Here's how the part is built. I have some questions about the finished solid (model axes, mm). Face numbers are marked on the shaded views. A direction names the side the tool comes from. Round coordinates to 2 decimals unless told otherwise and drop trailing zeros. Loops run counter-clockwise (first coordinate to the right, second up) from the corner with the lowest first, then second, coordinate; pieces in that order, holes last. Notation, with made-up numbers: M 6.25,43 L 16.25,43 A25 cw 16.25,78 Z; hole C 3.5,65.25 d5. An arc over 180 degrees is marked long. Answer as CSV lines item,"result".
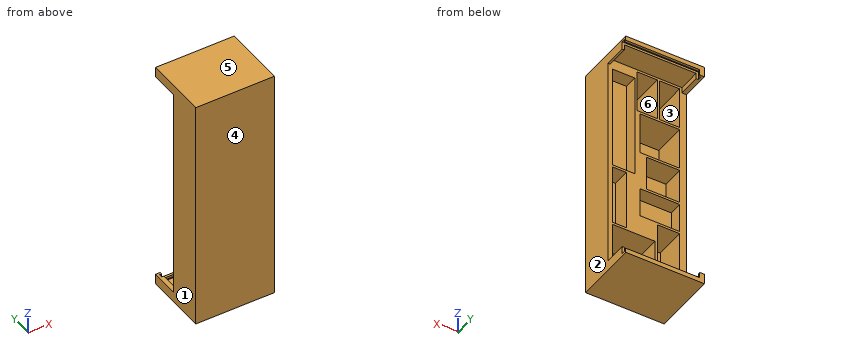
```python
from build123d import *

# Parameters (mm, degrees)
SKETCH1_4_W          = 19.5
SKETCH1_4_H          = 56.2
BOSS_EXTRUDE3_DEPTH  = 2
SKETCH1_5_W          = 12.1
SKETCH1_5_H          = 52.7
BOSS_EXTRUDE4_DEPTH  = 13.8
SKETCH1_W            = 19.5
SKETCH1_H            = 91.3
BOSS_EXTRUDE5_DEPTH  = 17.3
SKETCH1_8_W          = 34.6
SKETCH1_8_H          = 25.8
BOSS_EXTRUDE7_DEPTH  = 17.2
SKETCH1_9_W          = 28.8
SKETCH1_9_H          = 30.5
BOSS_EXTRUDE8_DEPTH  = 9.7
SKETCH1_10_W         = 17.5
SKETCH1_10_H         = 36.9
SKETCH1_10_W_2       = 28.8
SKETCH1_10_H_2       = 30.5
SKETCH1_10_W_3       = 34.6
SKETCH1_10_H_3       = 25.8
SKETCH1_10_W_4       = 19.5
SKETCH1_10_H_4       = 56.2
SKETCH1_10_W_5       = 12.1
SKETCH1_10_H_5       = 52.7
SKETCH1_10_W_6       = 37
SKETCH1_10_H_6       = 39.55
BOSS_EXTRUDE9_DEPTH  = 28.791978309
BOSS_EXTRUDE10_DEPTH = 48.4
BOSS_EXTRUDE11_DEPTH = 53.4
BOSS_EXTRUDE12_DEPTH = 2
SKETCH1_13_W         = 68.5
SKETCH1_13_H         = 206.3
BOSS_EXTRUDE13_DEPTH = 2


with BuildPart() as part:
    # Sketch1_4 → Boss-Extrude3 (new body)
    with BuildSketch(Plane(origin=(0, 0, 0), x_dir=(1, 0, 0), z_dir=(0, 1, 0))):
        with Locations((-18.5, 69.05)):
            Rectangle(SKETCH1_4_W, SKETCH1_4_H)
    extrude(amount=BOSS_EXTRUDE3_DEPTH)



with BuildPart() as body_2:
    # Sketch1_5 → Boss-Extrude4 (new body)
    with BuildSketch(Plane(origin=(0, 0, 0), x_dir=(1, 0, 0), z_dir=(0, 1, 0))):
        with Locations((24.2, 29.25)):
            Rectangle(SKETCH1_5_W, SKETCH1_5_H)
    extrude(amount=BOSS_EXTRUDE4_DEPTH)


with BuildPart() as body_3:
    # Sketch1 → Boss-Extrude5 (new body)
    with BuildSketch(Plane(origin=(0, 0, 0), x_dir=(1, 0, 0), z_dir=(0, 1, 0))):
        with Locations((20.5, -44.75)):
            Rectangle(SKETCH1_W, SKETCH1_H)
    extrude(amount=BOSS_EXTRUDE5_DEPTH)


with BuildPart() as body_4:
    # Sketch1_8 → Boss-Extrude7 (new body)
    with BuildSketch(Plane(origin=(0, 0, 0), x_dir=(1, 0, 0), z_dir=(0, 1, 0))):
        with Locations((-10.95, 26.05)):
            Rectangle(SKETCH1_8_W, SKETCH1_8_H)
    extrude(amount=BOSS_EXTRUDE7_DEPTH)


with BuildPart() as body_5:
    # Sketch1_9 → Boss-Extrude8 (new body)
    with BuildSketch(Plane(origin=(0, 0, 0), x_dir=(1, 0, 0), z_dir=(0, 1, 0))):
        with Locations((-13.85, -4.1)):
            Rectangle(SKETCH1_9_W, SKETCH1_9_H)
    extrude(amount=BOSS_EXTRUDE8_DEPTH)


with BuildPart() as part_1:
    add(part.part)

    add(body_2.part)  # Boss-Extrude9 merges body 2

    add(body_3.part)  # Boss-Extrude9 merges body 3

    add(body_4.part)  # Boss-Extrude9 merges body 4

    add(body_5.part)  # Boss-Extrude9 merges body 5
    # Sketch1_10 → Boss-Extrude9 (add)
    with BuildSketch(Plane(origin=(0, 0, 0), x_dir=(1, 0, 0), z_dir=(0, 1, 0))):
        Polygon((34.25, -94.15), (34.25, 94.15), (32.25, 94.15), (32.25, 99.15), (-30.25, 99.15), (-30.25, 94.15), (-34.25, 94.15), (-34.25, -94.15), (-30.25, -94.15), (-30.25, -99.15), (32.25, -99.15), (32.25, -94.15), align=None)
        with Locations((-19.5, -78.7)):
            Rectangle(SKETCH1_10_W, SKETCH1_10_H, mode=Mode.SUBTRACT)
        with Locations((0, -78.7)):
            Rectangle(SKETCH1_10_W, SKETCH1_10_H, mode=Mode.SUBTRACT)
        with Locations((-13.85, -4.1)):
            Rectangle(SKETCH1_10_W_2, SKETCH1_10_H_2, mode=Mode.SUBTRACT)
        with Locations((-10.95, -39.8)):
            Rectangle(SKETCH1_10_W_3, SKETCH1_10_H, mode=Mode.SUBTRACT)
        Polygon((29.25, -90.4), (10.75, -90.4), (10.75, 0.9), (30.25, 0.9), (30.25, -90.4), align=None, mode=Mode.SUBTRACT)
        with Locations((-10.95, 26.05)):
            Rectangle(SKETCH1_10_W_3, SKETCH1_10_H_3, mode=Mode.SUBTRACT)
        with Locations((-18.5, 69.05)):
            Rectangle(SKETCH1_10_W_4, SKETCH1_10_H_4, mode=Mode.SUBTRACT)
        with Locations((24.2, 29.25)):
            Rectangle(SKETCH1_10_W_5, SKETCH1_10_H_5, mode=Mode.SUBTRACT)
        with Locations((11.75, 77.375)):
            Rectangle(SKETCH1_10_W_6, SKETCH1_10_H_6, mode=Mode.SUBTRACT)
    extrude(amount=BOSS_EXTRUDE9_DEPTH)

    # Sketch1_11 → Boss-Extrude10 (add)
    with BuildSketch(Plane(origin=(0, 0, 0), x_dir=(1, 0, 0), z_dir=(0, 1, 0))):
        Polygon((34.25, -101.15), (34.25, -94.15), (32.25, -94.15), (32.25, -99.15), (-30.25, -99.15), (-30.25, -94.15), (-32.25, -94.15), (-32.25, -101.15), align=None)
        Polygon((34.25, 94.15), (34.25, 101.15), (-32.25, 101.15), (-32.25, 94.15), (-30.25, 94.15), (-30.25, 99.15), (32.25, 99.15), (32.25, 94.15), align=None)
    extrude(amount=BOSS_EXTRUDE10_DEPTH)

    # Sketch1_12 → Boss-Extrude11 (add)
    with BuildSketch(Plane(origin=(0, 0, 0), x_dir=(1, 0, 0), z_dir=(0, 1, 0))):
        Polygon((-32.25, -101.15), (-32.25, -94.15), (-34.25, -94.15), (-34.25, -103.15), (34.25, -103.15), (34.25, -101.15), align=None)
        Polygon((-32.25, 101.15), (34.25, 101.15), (34.25, 103.15), (-34.25, 103.15), (-34.25, 94.15), (-32.25, 94.15), align=None)
    extrude(amount=BOSS_EXTRUDE11_DEPTH)

    # Sketch2 → Boss-Extrude12 (add)
    with BuildSketch(Plane(origin=(0, 53.4, 0), x_dir=(1, 0, 0), z_dir=(0, 1, 0))):
        Polygon((-32.25, -94.15), (-32.25, -101.15), (34.25, -101.15), (34.25, -99.15), (-30.25, -99.15), (-30.25, -94.15), align=None)
        Polygon((-32.25, 94.15), (-32.25, 101.15), (34.25, 101.15), (34.25, 99.15), (-30.25, 99.15), (-30.25, 94.15), align=None)
    extrude(amount=-BOSS_EXTRUDE12_DEPTH)

    # Sketch1_13 → Boss-Extrude13 (add)
    with BuildSketch(Plane(origin=(0, 0, 0), x_dir=(1, 0, 0), z_dir=(0, 1, 0))):
        Rectangle(SKETCH1_13_W, SKETCH1_13_H)
    extrude(amount=-BOSS_EXTRUDE13_DEPTH)


solid = part_1.part
```
1. We'd pull the mould along X, two halves only. Please class the marked faces 1, 2, 3 and 4: pulls with the +X half, pulls with the -X half, needs draft (parallel to the pull), parting line crosses it, or undercut.
Evaluation:
face 1,"pulls with the -X half"
face 2,"pulls with the +X half"
face 3,"undercut"
face 4,"needs draft"
2. If I drill on line 1 (X direction, y = 3, z = 68.5); line 2 (Z direction, x = 23, y = 20); line 3 (X direction, y = 19.5, z = -25), over which ranges is the centre line in solid material (lowest first)? Write a range as [from, to].
Evaluation:
line 1,"x = [-34.25, -28.25], [-10.75, -8.75], [8.75, 34.25]"
line 2,"z = [-103.15, -97.15], [-57.6, -55.6], [-2.9, -0.9], [90.4, 103.15]"
line 3,"x = [-34.25, -28.25], [6.35, 18.15], [30.25, 34.25]"
3. I want a section at C-C, the plane z = 5.5. Please give me the cut outline in (x, y).
Evaluation:
outline,"M -34.25,-2 L 34.25,-2 L 34.25,28.79 L 30.25,28.79 L 30.25,17.3 L 10.75,17.3 L 10.75,28.79 L 0.55,28.79 L 0.55,9.7 L -28.25,9.7 L -28.25,28.79 L -34.25,28.79 Z"
4. I want a section at B-B, the plane y = 33.5. Please give me the cut outline in (x, z).
Evaluation:
outline,"M -34.25,-103.15 L 34.25,-103.15 L 34.25,-94.15 L 32.25,-94.15 L 32.25,-99.15 L -30.25,-99.15 L -30.25,-94.15 L -34.25,-94.15 Z; M -34.25,94.15 L -30.25,94.15 L -30.25,99.15 L 32.25,99.15 L 32.25,94.15 L 34.25,94.15 L 34.25,103.15 L -34.25,103.15 Z"
5. Which directions (+Z, -Z, +X, -X, +Y, -Y) give clear straight access to the entire face, cutting with the end or side of a thin tool? Please do the marked faces 5 and 6.
Evaluation:
face 5,"+Z, +X, -X, +Y, -Y"
face 6,"+Y"
6. I want a section at A-A, the plane y = 11.5. Please give me the cut outline in (x, z), and give its area (3 significant figures).
Evaluation:
outline,"M -34.25,-103.15 L 34.25,-103.15 L 34.25,103.15 L -34.25,103.15 Z; hole M -28.25,-97.15 L -8.75,-97.15 L -8.75,-40.95 L -28.25,-40.95 Z; hole M -28.25,-11.15 L 0.55,-11.15 L 0.55,19.35 L -28.25,19.35 Z; hole M -28.25,21.35 L 6.35,21.35 L 6.35,58.25 L -28.25,58.25 Z; hole M -28.25,60.25 L -10.75,60.25 L -10.75,97.15 L -28.25,97.15 Z; hole M -8.75,60.25 L 8.75,60.25 L 8.75,97.15 L -8.75,97.15 Z; hole M -6.75,-97.15 L 30.25,-97.15 L 30.25,-57.6 L -6.75,-57.6 Z"
area,"8,130 mm²"
7. For P1, Ø1.5, axis at x = -7.5, z = 73, coming from the +Y side; P2, Ø4, axis at x = 24, z = -20, coming from the +Y side, each with a flat end and sliding along its axis, tell me the tip position at first contact or that it passes through.
Evaluation:
P1,"stops at y = 0"
P2,"stops at y = 13.8"
